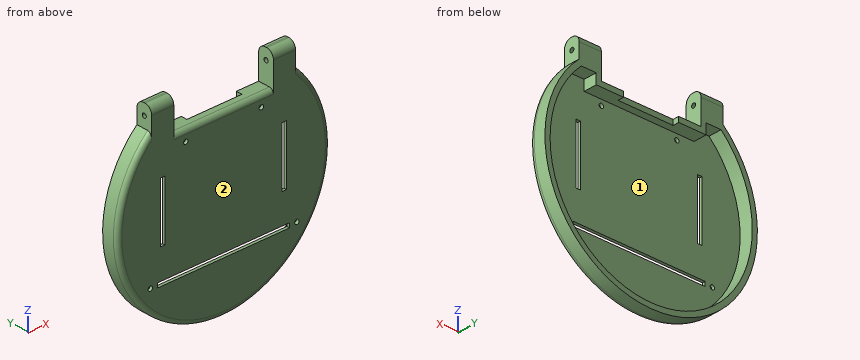
from build123d import *

# Parameters (mm, degrees)
SKETCH1_R           = 1.5
SKETCH1_W           = 90
SKETCH1_H           = 3
SKETCH1_W_2         = 3
SKETCH1_H_2         = 40
BOSS_EXTRUDE1_DEPTH = 2
BOSS_EXTRUDE2_DEPTH = 11
SKETCH3_W           = 15.108365525
SKETCH3_H           = 11
BOSS_EXTRUDE3_DEPTH = 15
SKETCH4_R           = 1.5
CUT_EXTRUDE1_DEPTH  = 115
FILLET2_R           = 3
FILLET3_R           = 5
SKETCH5_W           = 37.563728852
SKETCH5_H           = 8.292532788
CUT_EXTRUDE2_DEPTH  = 10


with BuildPart() as part:
    # Sketch1 → Boss-Extrude1 (new body)
    with BuildSketch(Plane(origin=(0, 0, 0), x_dir=(1, 0, 0), z_dir=(0, 1, 0))):
        with BuildLine():
            Line((-49.108365525, -55.238537207), (-34, -55.238537207))
            Line((-34, -55.238537207), (-34, -48.239677752))
            Line((-34, -48.239677752), (34, -48.239677752))
            Line((34, -48.239677752), (34, -55.238537207))
            Line((34, -55.238537207), (49.108365525, -55.238537207))
            ThreePointArc((49.108365525, -55.238537207), (0, 70.596427268), (-49.108365525, -55.238537207))
        make_face()
        with Locations(Location((-50, 34.976642786, 0), (0, 0, 270))):
            Circle(SKETCH1_R, mode=Mode.SUBTRACT)
        with Locations(Location((50, 34.976642786, 0), (0, 0, 270))):
            Circle(SKETCH1_R, mode=Mode.SUBTRACT)
        with Locations(Location((25.778764693, -40.884208467, 0), (0, 0, 270))):
            Circle(SKETCH1_R, mode=Mode.SUBTRACT)
        with Locations(Location((-25.778764696, -40.884208465, 0), (0, 0, 270))):
            Circle(SKETCH1_R, mode=Mode.SUBTRACT)
        with Locations((0, 34.976642786)):
            Rectangle(SKETCH1_W, SKETCH1_H, mode=Mode.SUBTRACT)
        with Locations((-41.5, -6.523357214)):
            Rectangle(SKETCH1_W_2, SKETCH1_H_2, mode=Mode.SUBTRACT)
        with Locations((41.5, -6.523357214)):
            Rectangle(SKETCH1_W_2, SKETCH1_H_2, mode=Mode.SUBTRACT)
    extrude(amount=BOSS_EXTRUDE1_DEPTH)

    # Sketch1_3 → Boss-Extrude2 (add)
    with BuildSketch(Plane(origin=(0, 0, 0), x_dir=(1, 0, 0), z_dir=(0, 1, 0))):
        with BuildLine():
            ThreePointArc((49.108365525, -55.238537207), (0, 70.596427268), (-49.108365525, -55.238537207))
            Line((-49.108365525, -55.238537207), (-34, -55.238537207))
            Line((-34, -55.238537207), (-34, -48.239677752))
            Line((-34, -48.239677752), (34, -48.239677752))
            Line((34, -48.239677752), (34, -55.238537207))
            Line((34, -55.238537207), (49.108365525, -55.238537207))
        make_face()
        with BuildLine():
            Line((-37.5, -51.738537207), (-47.722911854, -51.738537207))
            ThreePointArc((-47.722911854, -51.738537207), (0, 67.096427268), (47.722911854, -51.738537207))
            Line((47.722911854, -51.738537207), (37.5, -51.738537207))
            Line((37.5, -51.738537207), (37.5, -44.739677752))
            Line((37.5, -44.739677752), (-37.5, -44.739677752))
            Line((-37.5, -44.739677752), (-37.5, -51.738537207))
        make_face(mode=Mode.SUBTRACT)
    extrude(amount=BOSS_EXTRUDE2_DEPTH)

    # Sketch3 → Boss-Extrude3 (add)
    with BuildSketch(Plane.XY.offset(55.238537207)):
        with Locations((41.554182763, 5.5)):
            Rectangle(SKETCH3_W, SKETCH3_H)
        with Locations((-41.554182763, 5.5)):
            Rectangle(SKETCH3_W, SKETCH3_H)
    extrude(amount=BOSS_EXTRUDE3_DEPTH)

    # Sketch4 → Cut-Extrude1 (cut)
    with BuildSketch(Plane.ZY.offset(49.108365525)):
        with Locations((62.738537207, 5.5)):
            Circle(SKETCH4_R)
    extrude(amount=-CUT_EXTRUDE1_DEPTH, mode=Mode.SUBTRACT)

    # Fillet2
    fillet2_edges = [part.edges().sort_by_distance(p)[0] for p in [
        (0, 0, 48.239677752),
        (0, 0, -70.596427268),
    ]]
    fillet(fillet2_edges, radius=FILLET2_R)

    # Fillet3
    fillet3_edges = [part.edges().sort_by_distance(p)[0] for p in [
        (41.554182762, 0, 70.238537207),
        (41.554182762, 11, 70.238537207),
        (-41.554182762, 0, 70.238537207),
        (-41.554182762, 11, 70.238537207),
    ]]
    fillet(fillet3_edges, radius=FILLET3_R)

    # Sketch5 → Cut-Extrude2 (cut)
    with BuildSketch(Plane.XY.offset(48.239677752)):
        with Locations((0, 11)):
            Rectangle(SKETCH5_W, SKETCH5_H)
    extrude(amount=-CUT_EXTRUDE2_DEPTH, mode=Mode.SUBTRACT)


solid = part.part
Can you work these out from the model? Positions are in its coordinate system, mm. Face numbers are marked on the shaded views. Coordinates: 2 decimals unless noted, no trailing zeros. Order: outer loops, then holes, each group sorted by start corner. A loop starts at its lowest first (then second) coordinate and runs counter-clockwise, first axis right, second up. Notation, with made-up numbers: (0, 84) - (23, 84) arc R23 ccw to (23, 98) - close; hole circle Ø6 at (62.25, -9.75). An arc over 180 degrees is marked (long way). Answer as a JSON object with one key per item and string values. Group by question number.
Q1. I need wall thicknesses on line 1 (Z direction, x = 39, y = 5.25); line 2 (X direction, y = 10.25, z = 60.5); line 3 (Y direction, x = 58, z = 17.5). Which ranges of each line are inside material? Lowest first, please. Write a range as from..to.
Q2. Imagine slicing it at A-A (x = 0). Please give me the cut outline in (y, z).
Q3. Imagine slicing it at B-B (z = 14). Give the number of separate pieces and of enclosed holes in the cut face, and give its area (3 significant figures).
Q4. Will these pins go through, and if not, where does the flat tip stop? P1, Ø1, axis at x = 7, z = 47, coming from the +Y side; P2, Ø2.5, axis at x = 7, y = 5, coming from the -Z side; P3, Ø1.5, axis at x = -8.5, y = 8.5, coming from the +Z side.
Q5. We'd pull the mould along Z, two halves only. Please class the marked faces 1 and 2: +Z half, -Z half, draft (parallel to the pull), parting line (faces both ways), or undercut.
Determined:
{
 "1": {"line 1": "z = -59.21..-55.02, 51.74..61.26, 64.22..70.24", "line 2": "x = -49.11..-34, 34..49.11", "line 3": "y = 0..2"},
 "2": {"outline": "(0, -67.6) arc R3 ccw to (3, -70.6) - (11, -70.6) - (11, -67.1) - (2, -67.1) - (2, -36.48) - (0, -36.48) - close; (0, -33.48) - (2, -33.48) - (2, 44.74) - (6.85, 44.74) - (6.85, 48.24) - (3, 48.24) arc R3 ccw to (0, 45.24) - close"},
 "3": {"separate pieces": "3", "enclosed holes": "0", "area": "334 mm2"},
 "4": {"P1": "stops at y = 6.85", "P2": "stops at z = -70.37", "P3": "stops at z = -66.47"},
 "5": {"face 1": "undercut", "face 2": "draft"}
}
